Check sheet for the drawn part. Datum: minimum x, y, z corner. Units: mm. Coordinates: 2 decimals unless noted, no trailing zeros. Loops run counter-clockwise (first coordinate to the right, second up) from the corner with the lowest first, then second, coordinate; pieces in that order, holes last. Notation, with made-up numbers: (56, 38.25) -> (62, 38.25) arc R23 cw to (62, 52.25) -> close; hole circle Ø9 at (-5, 57.5). An arc over 180 degrees is marked (long way). Use CSV: the item, a comma, the result in double quotes. Start each with the question number.
1. Sectioned sample at C-C, the plane z = 0.85. Record the cut outline in (x, y) (3 decimals), and give its area (3 significant figures).
2. Sectioned sample at D-D, the plane x = 13.75. Record the cut outline in (y, z), and give its area (3 significant figures).
3. Gauge pin test, flat ends, axial feed: pin 1 (1.2 mm diameter, centred on x = 8, z = 0.5, fed in from +Y) (3 decimals); pin 2 (0.7 mm diameter, centred on x = 7, z = 1, fed in from -Y) (3 decimals). Record the tip position at first contact, or that the pin passes through.
4. Sectioned sample at A-A, the plane y = 14. Record the cut outline in (x, z) (3 decimals), and give its area (3 significant figures).
5. Thickness scan on L1, parallel to Z at x = 4.75, y = 5.75; L2, parallel to X at y = 10, z = 0.45 (3 decimals); L3, parallel to Y at x = 7.5, z = 1.3 (3 decimals). Record the ranges inside material, lowest first.
6. Sectioned sample at B-B, the plane x = 7. Record the cut outline in (y, z) (3 decimals).
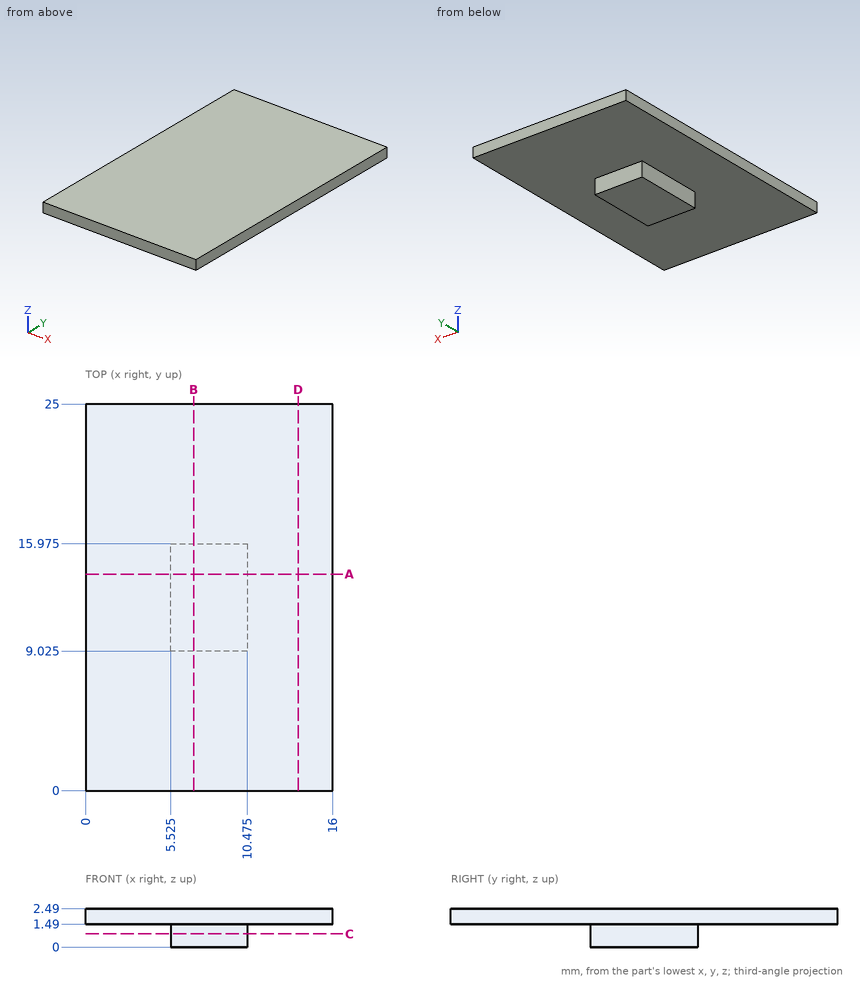
Completed:
1,outline,"(5.525, 9.025) -> (10.475, 9.025) -> (10.475, 15.975) -> (5.525, 15.975) -> close"
1,area,"34.4 mm²"
2,outline,"(0, 1.49) -> (25, 1.49) -> (25, 2.49) -> (0, 2.49) -> close"
2,area,"25.0 mm²"
3,pin 1,"y = 15.975"
3,pin 2,"y = 9.025"
4,outline,"(0, 1.49) -> (5.525, 1.49) -> (5.525, 0) -> (10.475, 0) -> (10.475, 1.49) -> (16, 1.49) -> (16, 2.49) -> (0, 2.49) -> close"
4,area,"23.4 mm²"
5,L1,"1.49 to 2.49"
5,L2,"5.525 to 10.475"
5,L3,"9.025 to 15.975"
6,outline,"(0, 1.49) -> (9.025, 1.49) -> (9.025, 0) -> (15.975, 0) -> (15.975, 1.49) -> (25, 1.49) -> (25, 2.49) -> (0, 2.49) -> close"
